from build123d import *

# Parameters (mm, degrees)
SKETCH_1_R          = 2.5
EXTRUDE_1_DEPTH     = 4
EXTRUDE_2_DEPTH     = 4
CUT_EXTRUDE_1_DEPTH = 5


with BuildPart() as part:
    # 草图1 → 凸台-拉伸1 (new body)
    with BuildSketch(Plane(origin=(0, 0, 0), x_dir=(1, 0, 0), z_dir=(0, 1, 0))):
        with BuildLine():
            Line((-55, 6), (55, 6))
            ThreePointArc((55, 6), (61, 0), (55, -6))
            Line((55, -6), (-55, -6))
            ThreePointArc((-55, -6), (-61, 0), (-55, 6))
        make_face()
        with Locations(Location((55, 0, 0), (0, 0, 270))):
            Circle(SKETCH_1_R, mode=Mode.SUBTRACT)
        with Locations(Location((-55, 0, 0), (0, 0, 270))):
            Circle(SKETCH_1_R, mode=Mode.SUBTRACT)
    extrude(amount=EXTRUDE_1_DEPTH)

    # 草图2 → 凸台-拉伸2 (add)
    with BuildSketch(Plane(origin=(0, 4, 0), x_dir=(1, 0, 0), z_dir=(0, 1, 0))):
        with BuildLine():
            Line((-6, -11), (-6, 11))
            ThreePointArc((-6, 11), (0, 17), (6, 11))
            Line((6, 11), (6, -11))
            ThreePointArc((6, -11), (0, -17), (-6, -11))
        make_face()
    extrude(amount=-EXTRUDE_2_DEPTH)

    # 草图3 → 切除-拉伸1 (cut)
    with BuildSketch(Plane(origin=(0, 4, 0), x_dir=(1, 0, 0), z_dir=(0, 1, 0))):
        with BuildLine():
            Line((-2.55, -11), (-2.55, 11))
            ThreePointArc((-2.55, 11), (0, 13.55), (2.55, 11))
            Line((2.55, 11), (2.55, -11))
            ThreePointArc((2.55, -11), (0, -13.55), (-2.55, -11))
        make_face()
    extrude(amount=-CUT_EXTRUDE_1_DEPTH, mode=Mode.SUBTRACT)


solid = part.part
Design review of the part built by this model. Coordinates are the model's own, in mm. A direction names the side the tool comes from. Coordinates: 2 decimals unless noted, no trailing zeros. Order: outer loops, then holes, each group sorted by start corner. A loop starts at its lowest first (then second) coordinate and runs counter-clockwise, first axis right, second up. Notation, with made-up numbers: (61, -31.75) -> (84, -31.75) arc R30 cw to (84, 0.25) -> close; hole circle Ø9 at (36.5, 60). An arc over 180 degrees is marked (long way). Use one line per item in the form item = value. Start each with the question number.
(1) Insertion check: pin 1 (2 mm diameter, centred on y = 2, z = -4.5, fed in from +X); pin 2 (2 mm diameter, centred on y = 2.5, z = -8, fed in from +X); pin 3 (1.2 mm diameter, centred on x = 40, y = 1.5, fed in from +Z); pin 4 (4 mm diameter, centred on x = 55, z = 0, fed in from +Y). Each pin has a flat end and moves straight along its axis. Give the tip position at first contact, or say it passes through.
(2) The part is to be moulded in two halves that separate along X. For faces 4 (the flat face through (-6, 2, 9)), 5 (the flat face through (-30, 2, 6)), 6 (the flat face through (2.55, 2, 0)), say which applies: +X half, -X half, draft (parallel to the pull), parting line (faces both ways), or undercut.
(3) Add section C-C on x = 26. State the section outline as (y, z) points.
(4) Add section A-A on y = 2.75. State the section outline as (x, z) points.
(5) For faces 1 (the cylindrical face through (0.06, 2.03, 13.55)), 2 (the flat face through (30, 2, -6)), 3 (the flat face through (31, 2, 6)), list the 3-axis set-ups (+Z, -Z, +X, -X, +Y, -Y) from which the entire face can be reached by the end or side of a thin tool; tool diameter is ignored.
(6) For probe 1 along X at (y, z) = (2, 0); probe 2 along X at (y, z) = (2.85, 7); probe 3 along Z at (x, y) = (-10.5, 0.85), list the stretches that pass through material, from the lowest coordinate up.
(7) Add section B-B on z = 0. State the section outline as (x, y) points.
Answer block:
q1.pin_1 = 59.87
q1.pin_2 = 6
q1.pin_3 = 6
q1.pin_4 = through
q2.face_4 = -X half
q2.face_5 = draft
q2.face_6 = undercut
q3.outline = (0, -6) -> (4, -6) -> (4, 6) -> (0, 6) -> close
q4.outline = (-55, -6) -> (-6, -6) -> (-6, -11) arc R6 ccw to (6, -11) -> (6, -6) -> (55, -6) arc R6 ccw to (55, 6) -> (6, 6) -> (6, 11) arc R6 ccw to (-6, 11) -> (-6, 6) -> (-55, 6) arc R6 ccw to start; hole circle Ø5 at (-55, 0); hole (-2.55, -11) arc R2.55 ccw to (2.55, -11) -> (2.55, 11) arc R2.55 ccw to (-2.55, 11) -> close; hole circle Ø5 at (55, 0)
q5.face_1 = +Y, -Y
q5.face_2 = -Z, +X, +Y, -Y
q5.face_3 = +Z, +X, +Y, -Y
q6.probe_1 = -61 to -57.5, -52.5 to -2.55, 2.55 to 52.5, 57.5 to 61
q6.probe_2 = -6 to -2.55, 2.55 to 6
q6.probe_3 = -6 to 6
q7.outline = (-61, 0) -> (-57.5, 0) -> (-57.5, 4) -> (-61, 4) -> close; (-52.5, 0) -> (-2.55, 0) -> (-2.55, 4) -> (-52.5, 4) -> close; (2.55, 0) -> (52.5, 0) -> (52.5, 4) -> (2.55, 4) -> close; (57.5, 0) -> (61, 0) -> (61, 4) -> (57.5, 4) -> close
